Input: dimensioned drawing with shaded views. Units: mm. Origin: part minimum x, y, z. Give positions to 0.01 mm unless a question says otherwise; leave off trailing zeros. Order: outer loops, then holes, each group sorted by start corner. A loop starts at its lowest first (then second) coordinate and runs counter-clockwise, first axis right, second up. Notation, with made-up numbers: (-10, -7.5) - (10, -7.5) arc R20 ccw to (10, -2.5) - close; hole circle Ø9 at (74, 44). An arc over 180 degrees is marked (long way). Answer as CSV lines item,"result".
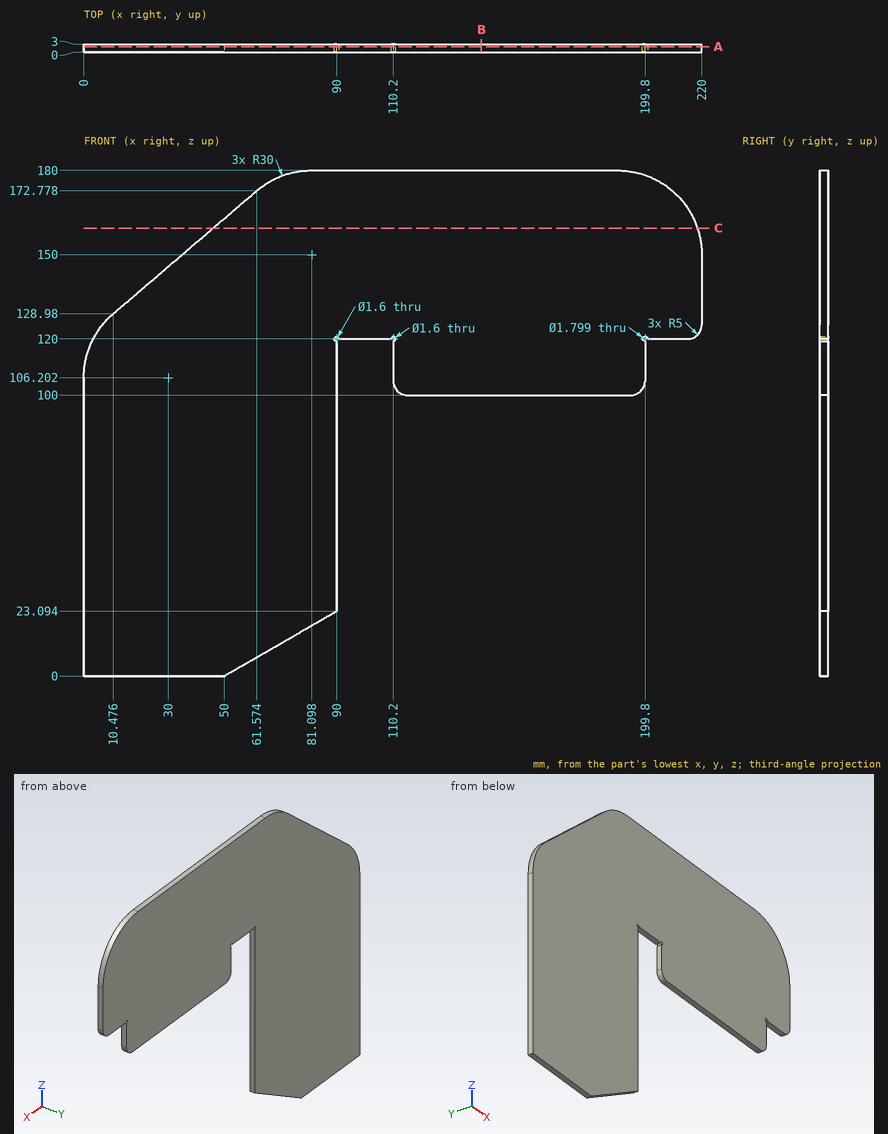
(1) Ray query, line 1 (X direction, y = 1.3, z = 86.5); line 2 (Z direction, x = 118.5, y = 1.7); line 3 (X direction, y = 0.9, z = 103). Return the intervals inside material, ascending. Write a range as from..to.
Completed:
line 1,"0..90"
line 2,"100..180"
line 3,"0..90, 110.62..199.38"
(2) Contact query for flat-ended pins moving along their axis: pin 1 (1.5 mm diameter, centred on x = 101.5, y = 1.5, fed in from -Z); pin 2 (1.4 mm diameter, centred on x = 90, z = 120, fed in from -Y); pin 3 (1.5 mm diameter, centred on x = 136, y = 1.5, fed in from -Z). Output: stop coordinate, or through.
Completed:
pin 1,"z = 120"
pin 2,"through"
pin 3,"z = 100"
(3) Cut plane A-A (y = 2.1). Return loops of the section in (x, z), then the cut area to 3 significant figures.
Completed:
outline,"(0, 0) - (50, 0) - (90, 23.09) - (90, 119.2) arc R0.8 cw (long way) to (90.8, 120) - (109.4, 120) arc R0.8 cw (long way) to (110.2, 119.2) - (110.2, 105) arc R5 ccw to (115.2, 100) - (194.8, 100) arc R5 ccw to (199.8, 105) - (199.8, 119.1) arc R0.9 cw (long way) to (200.7, 120) - (215, 120) arc R5 ccw to (220, 125) - (220, 150) arc R30 ccw to (190, 180) - (81.1, 180) arc R30 ccw to (61.57, 172.78) - (10.48, 128.98) arc R30 ccw to (0, 106.2) - close"
area,"23,000 mm²"
(4) Cut plane C-C (z = 159.5). Return loops of the section in (x, y).
Completed:
outline,"(46.08, 0) - (218.46, 0) - (218.46, 3) - (46.08, 3) - close"
(5) Cut plane B-B (x = 141.5). Return loops of the section in (y, z).
Completed:
outline,"(0, 100) - (3, 100) - (3, 180) - (0, 180) - close"
